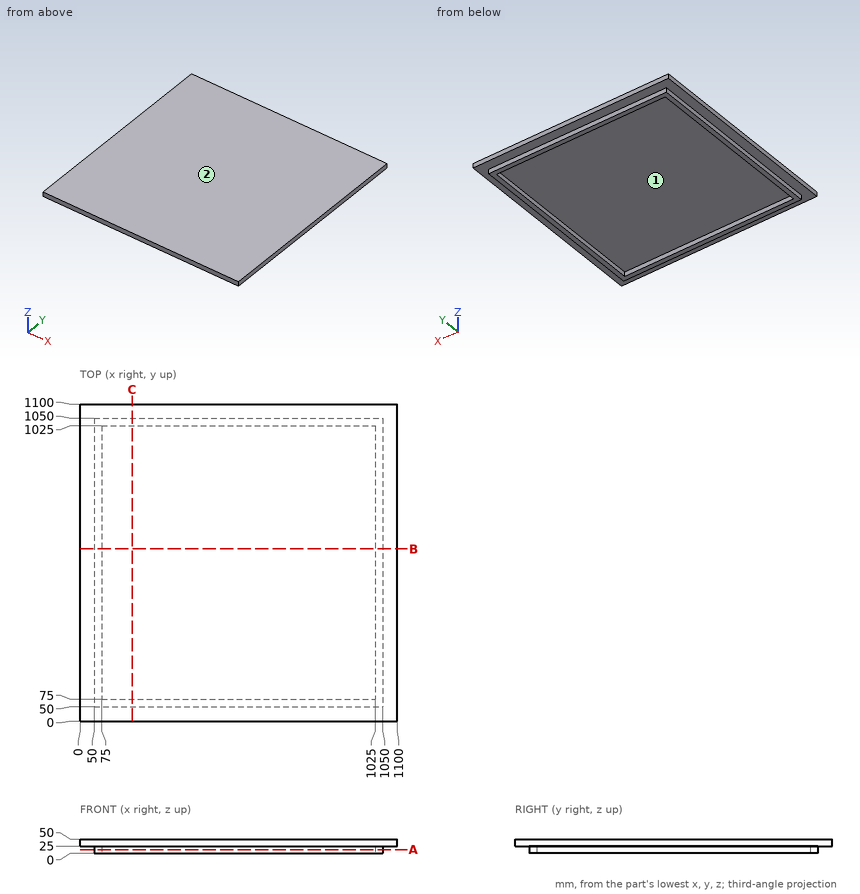
Can you work these out from the drawing? Everything is in mm from the part's minimum corner. Give positions to 0.01 mm unless a question says otherwise; leave off trailing zeros. Order: outer loops, then holes, each group sorted by start corner. A loop starts at its lowest first (then second) coordinate and runs counter-clockwise, first axis right, second up.
1. Will these pins go through, and if not, where does the flat tip stop? P1, Ø1, axis at y = 584.5, z = 12, coming from the +X side; P2, Ø12, axis at x = 895, z = 18, coming from the -Y side; P3, Ø10, axis at x = 570, y = 805, coming from the -Z side.
2. Suppose I cut it at B-B (y = 597.5). List the corners of the cut face in (x, z) for me, plus the area to 4 significant figures.
3. I need wall thicknesses on L1, parallel to Y at x = 81, z = 17; L2, parallel to Z at x = 671, y = 797.5. Which ranges of each line are inside material? Lowest first, please.
4. Suppose I cut it at A-A (z = 13). List the corners of the cut face in (x, y) for me, plus the area to 3 significant figures.
5. We'd pull the mould along X, two halves only. Please class the marked faces 1 and 2: pulls with the +X half, pulls with the -X half, needs draft (parallel to the pull), parting line crosses it, or undercut.
Solved:
1. P1: stops at x = 1050
1. P2: stops at y = 50
1. P3: stops at z = 25
2. outline: (0, 25) - (50, 25) - (50, 0) - (75, 0) - (75, 25) - (1025, 25) - (1025, 0) - (1050, 0) - (1050, 25) - (1100, 25) - (1100, 50) - (0, 50) - close
2. area: 28,750 mm2
3. L1: y = 50 to 75, 1025 to 1050
3. L2: z = 25 to 50
4. outline: (50, 50) - (1050, 50) - (1050, 1050) - (50, 1050) - close; hole (75, 75) - (1025, 75) - (1025, 1025) - (75, 1025) - close
4. area: 97,500 mm2
5. face 1: undercut
5. face 2: needs draft
